Autodesk Inventor part; units mm, degrees
ref_plane "YZ Plane" through (0, 0, 0) normal (1, 0, 0) x (0, 1, 0)
ref_plane "XZ Plane" through (0, 0, 0) normal (0, 1, 0) x (-1, 0, 0)
ref_plane "XY Plane" through (0, 0, 0) normal (0, 0, 1) x (1, 0, 0)
sketch "Esquisse1" plane through (0, 0, 0) normal (1, 0, 0) x (0, 1, 0)
  line L0 (0, 0) -> (0, -21.1525)
  line L1 (6, 0) -> (6, -40)
  line L2 (6.2, 0) -> (8, -4.9455)
  line L3 (8, -4.9455) -> (8, -40)
  line L4 (6, -40) -> (8, -40)
  line L5 (6, 0) -> (6.2, 0)
  dimension "d0" = 160
  dimension "d2" = 16
  dimension "d4" = 40
  dimension "d6" = 2
  dimension "d7" = 0.2
revolve "Révolution1" add sketch "Esquisse1" angle 360 about axis through (0, 0, 0) along (0, 0, -1)
chamfer "Chanfrein1" distance 0.5 angle 45 2 edges at (0, -6, -40) (0, -8, -40)
properties part number "douille" material "Aluminium 6061"
Design review of the part built by this model. Coordinates are the model's own, in mm. Coordinates: 2 decimals unless noted, no trailing zeros. Loops run counter-clockwise (first coordinate to the right, second up) from the corner with the lowest first, then second, coordinate; pieces in that order, holes last.
Item 1: Add section C-C (z = -6.5). Write out the cut boundary in (x, y), and give its area (3 significant figures).
Completed:
outline: circle Ø16 at (0, 0); hole circle Ø12 at (0, 0)
area: 88.0 mm2
Item 2: Draft analysis for pull direction Y (two halves, no side actions). For faces 1 (the flat face through (3, -6, -40)), 2 (the conical face through (-6.162, -1.368, -0.309)), 3 (the cylindrical face through (0, -6, -20)), state which applies: pulls with the +Y half, pulls with the -Y half, needs draft (parallel to the pull), parting line crosses it, or undercut.
Completed:
face 1: needs draft
face 2: parting line crosses it
face 3: undercut
Item 3: Wall thickness on L1, parallel to X at y = 0.25, z = -5; L2, parallel to Y at x = -3.25, z = -34; L3, parallel to X at y = -3.75, z = -5.5: over which ranges is each line inside the solid? List them lowest first.
Completed:
L1: x = -8 to -5.99, 5.99 to 8
L2: y = -7.31 to -5.04, 5.04 to 7.31
L3: x = -7.07 to -4.68, 4.68 to 7.07
Item 4: Add section A-A (y = 0). Write out the cut boundary in (x, z), and give its area (3 significant figures).
Completed:
outline: (-8, -39.5) - (-7.5, -40) - (-6.5, -40) - (-6, -39.5) - (-6, 0) - (-6.2, 0) - (-8, -4.95) - close; (6, -39.5) - (6.5, -40) - (7.5, -40) - (8, -39.5) - (8, -4.95) - (6.2, 0) - (6, 0) - close
area: 151 mm2
Item 5: Clearance check with flat-ended pins moving along their axes: pin 1 (3 mm diameter, centred on y = 2, z = -20, fed in from -X); pin 2 (1.5 mm diameter, centred on y = -4, z = -20, fed in from -X); pin 3 (6 mm diameter, centred on y = -5.5, z = -11.5, fed in from -X). State where each tip first meets the part, or that it passes through.
Completed:
pin 1: stops at x = -7.98
pin 2: stops at x = -7.31
pin 3: stops at x = -7.6
